Design review of the part built by this model. Coordinates are the model's own, in mm. Give positions to 0.01 mm unless a question says otherwise; leave off trailing zeros. Loops run counter-clockwise (first coordinate to the right, second up) from the corner with the lowest first, then second, coordinate; pieces in that order, holes last. Notation, with made-up numbers: M -33,-22.5 L 23,-22.5 A19 ccw 23,-10.5 Z; hole C 61,31 d6. An arc over 180 degrees is marked long. Answer as CSV lines item,"result".
```python
from build123d import *

# Parameters (mm, degrees)
SKETCH1_W           = 140
SKETCH1_H           = 140
BOSS_EXTRUDE1_DEPTH = 1
FILLET1_R           = 10
SKETCH2_R           = 2.1
CUT_EXTRUDE1_DEPTH  = 10


with BuildPart() as part:
    # Sketch1 → Boss-Extrude1 (new body)
    with BuildSketch(Plane(origin=(0, 0, 0), x_dir=(1, 0, 0), z_dir=(0, 1, 0))):
        with Locations((70, -70)):
            Rectangle(SKETCH1_W, SKETCH1_H)
    extrude(amount=BOSS_EXTRUDE1_DEPTH)

    # Fillet1
    fillet1_edges = [part.edges().sort_by_distance(p)[0] for p in [
        (0, 0.5, 0),
        (140, 0.5, 0),
        (140, 0.5, 140),
        (0, 0.5, 140),
    ]]
    fillet(fillet1_edges, radius=FILLET1_R)

    # Sketch2 → Cut-Extrude1 (cut)
    with BuildSketch(Plane(origin=(0, 1, 0), x_dir=(1, 0, 0), z_dir=(0, 1, 0))):
        with Locations(Location((98.75, -98.75, 0), (0, 0, 270))):
            Circle(SKETCH2_R)
        with Locations(Location((41.25, -98.75, 0), (0, 0, 270))):
            Circle(SKETCH2_R)
        with Locations(Location((41.25, -41.25, 0), (0, 0, 270))):
            Circle(SKETCH2_R)
        with Locations(Location((98.75, -41.25, 0), (0, 0, 270))):
            Circle(SKETCH2_R)
        with Locations(Location((72.15, -57.85, 0), (0, 0, 270))):
            Circle(SKETCH2_R)
        with Locations(Location((94.15, -57.85, 0), (0, 0, 270))):
            Circle(SKETCH2_R)
        with Locations(Location((72.15, -82.15, 0), (0, 0, 270))):
            Circle(SKETCH2_R)
        with Locations(Location((94.15, -82.15, 0), (0, 0, 270))):
            Circle(SKETCH2_R)
    extrude(amount=-CUT_EXTRUDE1_DEPTH, mode=Mode.SUBTRACT)


solid = part.part
```
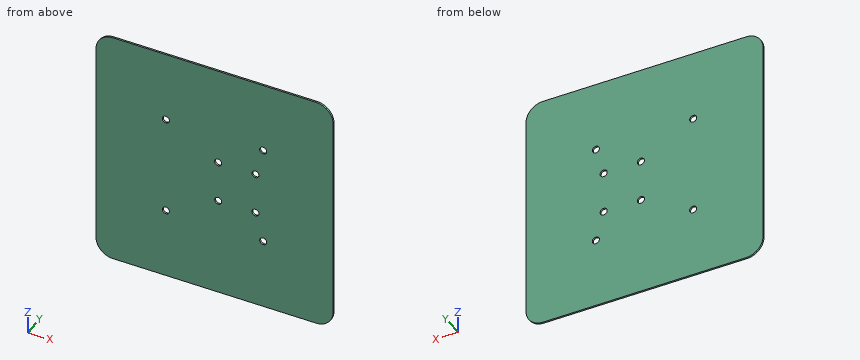
1. We need section A-A, the plane x = 98.75. Write out the cut boundary in (y, z).
Answer block:
outline,"M 0,0 L 1,0 L 1,39.15 L 0,39.15 Z; M 0,43.35 L 1,43.35 L 1,96.65 L 0,96.65 Z; M 0,100.85 L 1,100.85 L 1,140 L 0,140 Z"
2. We need section B-B, the plane z = 41.25. Write out the cut boundary in (x, y), plus the area to 3 significant figures.
Answer block:
outline,"M 0,0 L 39.15,0 L 39.15,1 L 0,1 Z; M 43.35,0 L 96.65,0 L 96.65,1 L 43.35,1 Z; M 100.85,0 L 140,0 L 140,1 L 100.85,1 Z"
area,"132 mm²"
3. To check wall thickness, follow L1, parallel to X at y = 0.45, z = 98.75; L2, parallel to Z at x = 41, y = 0.7; L3, parallel to X at y = 0.8, z = 57.85. State the ranges of each line that lie inside material, in increasing order. Write a range as [from, to].
Answer block:
L1,"[0, 39.15], [43.35, 96.65], [100.85, 140]"
L2,"[0, 39.16], [43.34, 96.66], [100.84, 140]"
L3,"[0, 70.05], [74.25, 92.05], [96.25, 140]"
4. For P1, Ø3, axis at x = 53, z = 77, coming from the -Y side, flat-tipped, find the tip position at first contact; note if it passes through.
Answer block:
P1,"y = 0"
